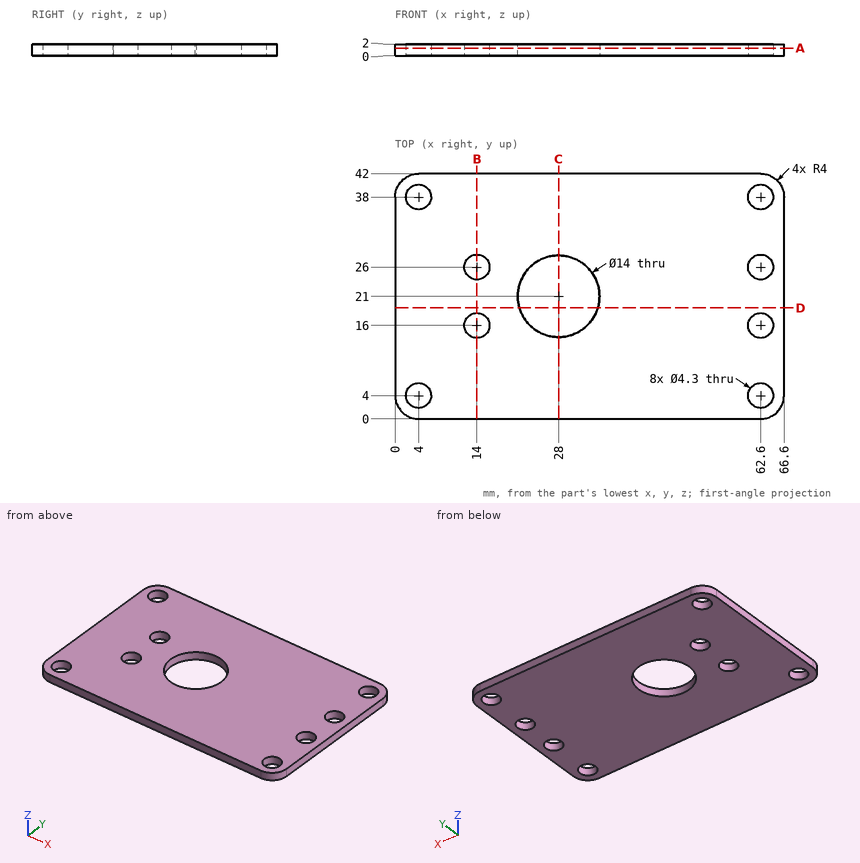
Part print with two shaded views. Sizes in mm from the minimum x, y, z corner. Round coordinates to 2 decimals unless told otherwise and drop trailing zeros. Loops run counter-clockwise (first coordinate to the right, second up) from the corner with the lowest first, then second, coordinate; pieces in that order, holes last. Notation, with made-up numbers: M 49,84.25 L 61,84.25 A18 cw 61,115.25 Z; hole C 69,27.5 d10. An arc over 180 degrees is marked long. Put each result on its own line as item: value. Start each with the question number.
Item 1: Cut at D-D (y = 19). List the corners of the cut face in (x, z).
Item 2: Drill centre lines: line 1 along Y through (x, z) = (62.6, 1.6); line 2 along X through (y, z) = (38, 0.55); line 3 along Y through (x, z) = (4, 0.5). Where is each one in solid material? Low to high.
Item 3: Cut at C-C (x = 28). List the corners of the cut face in (y, z).
Item 4: Cut at A-A (z = 1.3). Give the number of separate pieces and of enclosed holes in the cut face, then the cut area to 3 significant figures.
Item 5: Cut at B-B (x = 14). List the corners of the cut face in (y, z), then the cut area to 3 significant figures.
Item 6: Drop a flat-ended pin along its axis: P1, Ø3.5, axis at x = 62.6, y = 26, coming from the -Z side. Give the stop position or say it passes through.
Answer block:
1. outline: M 0,0 L 21.29,0 L 21.29,2 L 0,2 Z; M 34.71,0 L 66.6,0 L 66.6,2 L 34.71,2 Z
2. line 1: 0 to 1.85, 6.15 to 13.85, 18.15 to 23.85, 28.15 to 35.85, 40.15 to 42
2. line 2: 0 to 1.85, 6.15 to 60.45, 64.75 to 66.6
2. line 3: 0 to 1.85, 6.15 to 35.85, 40.15 to 42
3. outline: M 0,0 L 14,0 L 14,2 L 0,2 Z; M 28,0 L 42,0 L 42,2 L 28,2 Z
4. separate pieces: 1
4. enclosed holes: 9
4. area: 2,510 mm2
5. outline: M 0,0 L 13.85,0 L 13.85,2 L 0,2 Z; M 18.15,0 L 23.85,0 L 23.85,2 L 18.15,2 Z; M 28.15,0 L 42,0 L 42,2 L 28.15,2 Z
5. area: 66.8 mm2
6. P1: through
